Source: CAD feature listing. Evaluate the final solid. Frame: model axes, mm. A direction names the side the tool comes from. Round coordinates to 2 decimals unless told otherwise and drop trailing zeros. Loops run counter-clockwise (first coordinate to the right, second up) from the corner with the lowest first, then second, coordinate; pieces in that order, holes last. Notation, with made-up numbers: M -5,-36.5 L 45,-36.5 A21 cw 45,-3.5 Z; hole C 69,35 d10. An arc over 180 degrees is marked long. One line per item, written item: value.
from build123d import *

# Parameters (mm, degrees)
CHANFREIN1_SIZE = 0.3


with BuildPart() as part:
    # Esquisse1 → Révolution1 (revolve)
    with BuildSketch(Plane.XY, mode=Mode.PRIVATE) as r_volution1_sk:
        Polygon((36, 0), (36, 2), (31, 2), (31, 2.5), (-8, 2.5), (-8, 2), (-13, 2), (-13, 1.2), (0, 1.2), (0, 0), align=None)
    revolve(r_volution1_sk.sketch.rotate(Axis((-77.893994415, 0, 0), (1, 0, 0)), 90), axis=Axis((-77.893994415, 0, 0), (1, 0, 0)))

    # Chanfrein1
    chanfrein1_edges = [part.edges().sort_by_distance(p)[0] for p in [
        (36, 0, -2),
        (-8, 0, -2.5),
        (31, 0, -2.5),
    ]]
    chamfer(chanfrein1_edges, length=CHANFREIN1_SIZE)


solid = part.part
1. Section query A-A (y = 0). Return the cut outline in (x, z).
Report:
outline: M -13,-2 L -8,-2 L -8,-2.2 L -7.7,-2.5 L 30.7,-2.5 L 31,-2.2 L 31,-2 L 35.7,-2 L 36,-1.7 L 36,1.7 L 35.7,2 L 31,2 L 31,2.2 L 30.7,2.5 L -7.7,2.5 L -8,2.2 L -8,2 L -13,2 L -13,1.2 L 0,1.2 L 0,-1.2 L -13,-1.2 Z
2. Pin query (flat end, axial travel): pin 1 (1.5 mm diameter, centred on x = 11, y = -1, fed in from +Z); pin 2 (3 mm diameter, centred on x = 2.5, z = 0.5, fed in from +Y). Return the tip coordinate at first contact, or that it passes through.
Report:
pin 1: stops at z = 2.49
pin 2: stops at y = 2.5
3. Pull-direction query (Y, two-part tool) for faces 3 (the face through (33, 2, 0)), 4 (the face through (-13, 1, 1)), 5 (the face through (0, 0, 0)); classes: released by +Y, released by -Y, zero draft, split by the parting line, or undercut.
Report:
face 3: split by the parting line
face 4: zero draft
face 5: undercut
4. Section query D-D (x = 24). Return the cut outline in (y, z).
Report:
outline: C 0,0 d5
5. Section query B-B (x = -4). Return the cut outline in (y, z).
Report:
outline: C 0,0 d5; hole C 0,0 d2.4
6. Reachability of faces 1 (the face through (-6.41, -1.01, 0.65)), 2 (the face through (11.2, -0.1, -2.5)) from +Z, -Z, +X, -X, +Y, -Y: full face, straight path, thin tool, end or side. Return the list, or none.
Report:
face 1: -X
face 2: +X, -X
7. Ray query, line 1 (Y direction, x = -5, z = 0); line 2 (Y direction, x = -8.5, z = 0); line 3 (X direction, y = -0.75, z = 1.9). Return the intervals inside material, ascending. Write a range as [from, to].
Report:
line 1: y = [-2.5, -1.2], [1.2, 2.5]
line 2: y = [-2, -1.2], [1.2, 2]
line 3: x = [-8, 31]
